Build history of the part. All positions in model axes, mm. A direction names the side the tool comes from. Coordinates: 2 decimals unless noted, no trailing zeros. Loops run counter-clockwise (first coordinate to the right, second up) from the corner with the lowest first, then second, coordinate; pieces in that order, holes last.
(1) Slice it at D-D (z = 17.35). Give the cut face in (x, y).
(2) Wall check: L1, parallel to X at y = 0.85, z = 17.35; L2, parallel to Z at x = 11.6, y = 1.3; L3, parallel to X at y = 1.2, z = 17. Give the ranges that are in metal, low to high.
(3) Flat gauge pins, fed straight in: P1, Ø1.3, axis at x = -1, y = -1.5, coming from the +Z side; P2, Ø2, axis at x = -1.5, y = -2, coming from the -Z side; P3, Ø6, axis at x = 8.5, z = -10.5, coming from the -Y side. Where does each tip first touch, or does it go through?
(4) Slice it at A-A (z = -17.35). Give the cut face in (x, y), and give its area (3 significant figures).
(5) Tool access for faces 1 (the face through (-13.1, 2, 0)), 2 (the face through (0, 2, 15.05)), 3 (the face through (-8.89, -1, -18)): list every direction of +Z, -Z, +X, -X, +Y, -Y with a clear straight run to the whole face (end or side of a thin tool).
(6) Slice it at C-C (x = -0.5). Give the cut face in (y, z), and give its area (3 significant figures).
(7) Slice it at B-B (x = 11.6). Give the cut face in (y, z).
(8) Two-plate mould, pull along X, no slides. Class faces 4 (the face through (-13.9, 1, 0)), 5 (the face through (-11.74, 0.81, -18.44)), 6 (the face through (0, 1, -19.65)): pulls with the +X half, pulls with the -X half, needs draft (parallel to the pull), parting line crosses it, or undercut.
from build123d import *

# Parameters (mm, degrees)
SKETCH_1_W          = 27.8
SKETCH_1_H          = 39.3
EXTRUDE_1_DEPTH     = 1.6
SKETCH_2_R          = 1.1
CUT_EXTRUDE_1_DEPTH = 1.6
SKETCH_3_W          = 26.2
SKETCH_3_H          = 30.1
EXTRUDE_2_DEPTH     = 1.6
SKETCH_4_W          = 17.78
SKETCH_4_H          = 2.54
EXTRUDE_3_DEPTH     = 2.54


with BuildPart() as part:
    # 草图1 → 凸台-拉伸1 (new body)
    with BuildSketch(Plane(origin=(0, 0, 0), x_dir=(1, 0, 0), z_dir=(0, 1, 0))):
        Rectangle(SKETCH_1_W, SKETCH_1_H)
    extrude(amount=EXTRUDE_1_DEPTH)

    # 草图2 → 切除-拉伸1 (cut)
    with BuildSketch(Plane(origin=(0, 1.6, 0), x_dir=(1, 0, 0), z_dir=(0, 1, 0))):
        with Locations((-11.6, 17.35)):
            Circle(SKETCH_2_R)
        with Locations((11.6, 17.35)):
            Circle(SKETCH_2_R)
        with Locations((-11.6, -17.35)):
            Circle(SKETCH_2_R)
        with Locations((11.6, -17.35)):
            Circle(SKETCH_2_R)
    extrude(amount=-CUT_EXTRUDE_1_DEPTH, mode=Mode.SUBTRACT)

    # 草图3 → 凸台-拉伸2 (add)
    with BuildSketch(Plane(origin=(0, 1.6, 0), x_dir=(1, 0, 0), z_dir=(0, 1, 0))):
        Rectangle(SKETCH_3_W, SKETCH_3_H)
    extrude(amount=EXTRUDE_2_DEPTH)

    # 草图4 → 凸台-拉伸3 (add)
    with BuildSketch(Plane.XZ):
        with Locations((0, -17.68)):
            Rectangle(SKETCH_4_W, SKETCH_4_H)
    extrude(amount=EXTRUDE_3_DEPTH)


solid = part.part
Response values:
1. outline: (-13.9, 0) - (-12.7, 0) - (-12.7, 1.6) - (-13.9, 1.6) - close; (-10.5, 0) - (10.5, 0) - (10.5, 1.6) - (-10.5, 1.6) - close; (12.7, 0) - (13.9, 0) - (13.9, 1.6) - (12.7, 1.6) - close
2. L1: x = -13.9 to -12.7, -10.5 to 10.5, 12.7 to 13.9
2. L2: z = -19.65 to -18.45, -16.25 to 16.25, 18.45 to 19.65
2. L3: x = -13.9 to -12.64, -10.56 to 10.56, 12.64 to 13.9
3. P1: stops at z = -16.41
3. P2: stops at z = -18.95
3. P3: stops at y = 0
4. outline: (-13.9, 0) - (-12.7, 0) - (-12.7, 1.6) - (-13.9, 1.6) - close; (-10.5, 0) - (-8.89, 0) - (-8.89, -2.54) - (8.89, -2.54) - (8.89, 0) - (10.5, 0) - (10.5, 1.6) - (-10.5, 1.6) - close; (12.7, 0) - (13.9, 0) - (13.9, 1.6) - (12.7, 1.6) - close
4. area: 82.6 mm2
5. face 1: +Z, -Z, -X, +Y
5. face 2: +Z, +X, -X, +Y
5. face 3: +Z, -Z, -X, -Y
6. outline: (-2.54, -18.95) - (0, -18.95) - (0, -19.65) - (1.6, -19.65) - (1.6, -15.05) - (3.2, -15.05) - (3.2, 15.05) - (1.6, 15.05) - (1.6, 19.65) - (0, 19.65) - (0, -16.41) - (-2.54, -16.41) - close
6. area: 117 mm2
7. outline: (0, -19.65) - (1.6, -19.65) - (1.6, -18.45) - (0, -18.45) - close; (0, -16.25) - (1.6, -16.25) - (1.6, -15.05) - (3.2, -15.05) - (3.2, 15.05) - (1.6, 15.05) - (1.6, 16.25) - (0, 16.25) - close; (0, 18.45) - (1.6, 18.45) - (1.6, 19.65) - (0, 19.65) - close
8. face 4: pulls with the -X half
8. face 5: undercut
8. face 6: needs draft
